Build history of the part. All positions in model axes, mm. Face numbers are marked on the shaded views. A direction names the side the tool comes from. Coordinates: 2 decimals unless noted, no trailing zeros. Order: outer loops, then holes, each group sorted by start corner. A loop starts at its lowest first (then second) coordinate and runs counter-clockwise, first axis right, second up. Notation, with made-up numbers: M 43,50.25 L 67,50.25 A15 cw 67,69.25 Z; hole C -14,36 d3. An arc over 180 degrees is marked long. Write item = value, one per line. Start each with the question number.
Q1. 3-axis set-ups, long thin cutter, end or side, ignore diameter. For the marked faces 1, 2 and 3: which of +Z, -Z, +X, -X, +Y, -Y reach the whole face in a straight line?
Q2. Drill centre lines: probe 1 along Y at (x, z) = (-6, 7.5); probe 2 along X at (y, z) = (-10, 6.5). Where is each one in solid material? Low to high.
Q3. Band-saw the part on B-B on z = 0.75. Write the cut outline in (x, y), plus the area to 3 significant figures.
Q4. Band-saw the part on D-D on x = 14.5. Write the cut outline in (y, z), plus the area to 3 significant figures.
Q5. Band-saw the part on C-C on y = -3.5. Write the cut outline in (x, z), plus the area to 3 significant figures.
Q6. Pull direction X, two halves, no side cores. Call the marked faces 4, 5 and 6: released by +X, released by -X, zero draft, split by the parting line, or undercut.
Q7. Band-saw the part on A-A on x = 0. Write the cut outline in (y, z).
Q8. Pin check, flat tips, straight feed: P1, Ø1.5, axis at x = -15, z = 2, coming from the +Y side; P2, Ø2.5, axis at x = 8, y = -19.5, coming from the +Z side; P3, Ø1.4, axis at x = -17.5, y = -6.5, coming from the -Z side. Stop position of each tip, or through.
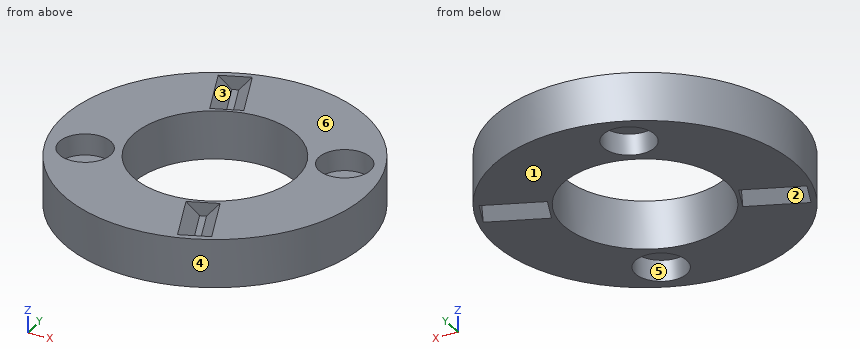
```python
from build123d import *

# Parameters (mm, degrees)
ESQUISSE1_R              = 25
ESQUISSE1_R_2            = 11
BOSS_EXTRU_1_DEPTH       = 8
ENL_V_START              = -14
ENL_V_MAT_EXTRU_9_DEPTH  = 10
ESQUISSE10_R             = 4.25
ENL_V_MAT_EXTRU_5_DEPTH  = 3.5
ESQUISSE12_R             = 4.25
ENL_V_MAT_EXTRU_6_DEPTH  = 3.5
ESQUISSE13_R             = 13.5
ENL_V_MAT_EXTRU_7_DEPTH  = 10
ENL_V_MAT_EXTRU_10_DEPTH = 10


with BuildPart() as part:
    # Esquisse1 → Boss.-Extru.1 (new body)
    with BuildSketch(Plane.XY):
        Circle(ESQUISSE1_R)
        Circle(ESQUISSE1_R_2, mode=Mode.SUBTRACT)
    extrude(amount=BOSS_EXTRU_1_DEPTH)

    # Esquisse16 → Enlèv. mat.-Extru.9 (cut)
    with BuildSketch(Plane(origin=(0, 0, 0), x_dir=(-0.9281017411356184, -0.3723266819622707, 0), z_dir=(-0.3723266819622707, 0.9281017411356184, 0)).offset(ENL_V_START)):
        Polygon((-2.5, 8), (2.5, 8), (0.5, 5.763932023), (-0.5, 5.763932023), align=None)
    enl_v_mat_extru_9 = extrude(amount=-ENL_V_MAT_EXTRU_9_DEPTH, mode=Mode.SUBTRACT)

    # Symétrie4: Enlèv. mat.-Extru.9 across plane
    add(enl_v_mat_extru_9.mirror(Plane(origin=(0, 0, 0), x_dir=(0, 0, 1), z_dir=(-0.3723266819622707, 0.9281017411356184, 0))), mode=Mode.SUBTRACT)

    # Esquisse10 → Enlèv. mat.-Extru.5 (cut)
    with BuildSketch(Plane(origin=(0, 0, 0), x_dir=(-1, 0, 0), z_dir=(0, 0, -1))):
        with Locations((7.074206957, 17.633933082)):
            Circle(ESQUISSE10_R)
        with Locations((-7.074206957, -17.633933082)):
            Circle(ESQUISSE10_R)
    extrude(amount=-ENL_V_MAT_EXTRU_5_DEPTH, mode=Mode.SUBTRACT)

    # Esquisse12 → Enlèv. mat.-Extru.6 (cut)
    with BuildSketch(Plane.XY.offset(8)):
        with Locations((17.633933082, 7.074206957)):
            Circle(ESQUISSE12_R)
        with Locations((-17.633933082, -7.074206957)):
            Circle(ESQUISSE12_R)
    extrude(amount=-ENL_V_MAT_EXTRU_6_DEPTH, mode=Mode.SUBTRACT)

    # Esquisse13 → Enlèv. mat.-Extru.7 (cut)
    with BuildSketch(Plane.XY.offset(8)):
        Circle(ESQUISSE13_R)
    extrude(amount=-ENL_V_MAT_EXTRU_7_DEPTH, mode=Mode.SUBTRACT)

    # Esquisse18 → Enlèv. mat.-Extru.10 (cut)
    with BuildSketch(Plane(origin=(0, 0, 8), x_dir=(0, 0, 1), z_dir=(-0.9281017411356183, -0.37232668196227087, 0)).offset(ENL_V_START)):
        Polygon((-8, -2.5), (-8, 2.5), (-5.763932023, 0.5), (-5.763932023, -0.5), align=None)
    enl_v_mat_extru_10 = extrude(amount=-ENL_V_MAT_EXTRU_10_DEPTH, mode=Mode.SUBTRACT)

    # Symétrie5: Enlèv. mat.-Extru.10 across plane
    add(enl_v_mat_extru_10.mirror(Plane(origin=(0, 0, 8), x_dir=(0, 0, 1), z_dir=(-0.9281017411356183, -0.37232668196227087, 0))), mode=Mode.SUBTRACT)


solid = part.part
```
Recorded:
q1.face_1 = -Z, +X, -X, +Y, -Y
q1.face_2 = -Z
q1.face_3 = +Z
q2.probe_1 = -24.27 to -12.09, 12.09 to 12.68, 20.47 to 24.27
q2.probe_2 = -22.91 to -20.72, -14.55 to -9.07, 9.07 to 22.91
q3.outline = C 0,0 d50; hole M -22.96,-7.24 L -21.59,-10.63 L -12.31,-6.91 L -13.67,-3.51 Z; hole C 0,0 d27; hole C -7.07,17.63 d8.5; hole C 7.07,-17.63 d8.5; hole M 12.31,6.91 L 13.67,3.51 L 22.96,7.24 L 21.59,10.63 Z
q3.area = 1,200 mm2
q4.outline = M -20.37,0 L 3.12,0 L 5.28,2.24 L 6.36,2.24 L 8.51,0 L 20.37,0 L 20.37,8 L 9.94,8 L 9.94,4.5 L 4.2,4.5 L 4.2,8 L -20.37,8 Z
q4.area = 299 mm2
q5.outline = M -24.75,0 L -15.44,0 L -13.68,0.73 L -13.68,0 L -13.04,0 L -13.04,8 L -15.33,8 L -15.33,4.5 L -19.93,4.5 L -19.93,8 L -24.75,8 Z; M 13.04,0 L 24.75,0 L 24.75,8 L 13.04,8 Z
q5.area = 171 mm2
q6.face_4 = split by the parting line
q6.face_5 = undercut
q6.face_6 = zero draft
q7.outline = M -25,0 L -13.5,0 L -13.5,8 L -25,8 Z; M 13.5,0 L 25,0 L 25,8 L 13.5,8 Z
q8.P1 = 20.54
q8.P2 = 6.79
q8.P3 = 1.47
